from build123d import *

# Parameters (mm, degrees)
BOSS_EXTRUDE1_DEPTH = 5
SKETCH2_R           = 3
CUT_EXTRUDE1_DEPTH  = 5
CUT_EXTRUDE2_DEPTH  = 5
CUT_EXTRUDE7_DEPTH  = 5


with BuildPart() as part:
    # Sketch1 → Boss-Extrude1 (new body)
    with BuildSketch(Plane.XY):
        with BuildLine():
            Line((-0.6, -8), (-0.6, 192))
            Line((-0.6, 192), (11.4, 192))
            Line((11.4, 192), (11.4, -8))
            ThreePointArc((11.4, -8), (5.4, -14), (-0.6, -8))
        make_face()
    extrude(amount=BOSS_EXTRUDE1_DEPTH)

    # Sketch2 → Cut-Extrude1 (cut)
    with BuildSketch(Plane.XY.offset(5)):
        with Locations((5.4, -8)):
            Circle(SKETCH2_R)
    extrude(amount=-CUT_EXTRUDE1_DEPTH, mode=Mode.SUBTRACT)

    # Sketch4 → Cut-Extrude2 (cut)
    with BuildSketch(Plane.XY.offset(5)):
        with BuildLine():
            Line((2.4, 102), (2.4, 42))
            ThreePointArc((2.4, 42), (5.4, 39), (8.4, 42))
            Line((8.4, 42), (8.4, 102))
            ThreePointArc((8.4, 102), (5.4, 105), (2.4, 102))
        make_face()
    extrude(amount=-CUT_EXTRUDE2_DEPTH, mode=Mode.SUBTRACT)

    # Sketch5 → Cut-Extrude7 (cut)
    with BuildSketch(Plane.XY.offset(5)):
        with BuildLine():
            Line((2.4, 192), (2.4, 142))
            ThreePointArc((2.4, 142), (5.4, 139), (8.4, 142))
            Line((8.4, 142), (8.4, 192))
            Line((8.4, 192), (2.4, 192))
        make_face()
    extrude(amount=-CUT_EXTRUDE7_DEPTH, mode=Mode.SUBTRACT)


solid = part.part
Geometry: final body of the model. Coordinates: model frame, mm. A direction names the side the tool comes from. Give positions to 0.01 mm unless a question says otherwise; leave off trailing zeros. Write each loop counter-clockwise with the first axis right and the second up, starting at its lowest first coordinate (ties: lowest second). Pieces come first, ordered by that corner, then holes.
(1) Cut plane B-B, the plane x = 5.4. Return loops of the section in (y, z).
(2) Mould query, pull axis X, two halves, no side actions, for faces 1 (the flat face through (1, 90, 0)), 2 (the flat face through (2.4, 167, 3)), 3 (the flat face through (-0.6, 91, 2)), 4 (the cylindrical face through (5.3, 39, 2.5)). Classes: released by +X, released by -X, zero draft, split by the parting line, or undercut.
(3) First-contact query: P1, Ø1, axis at x = 3.5, z = 4, coming from the +Y side; P2, Ø6, axis at x = 4, y = 102, coming from the -Z side; P3, Ø1, axis at x = 9, z = 1.5, coming from the -Y side. Flat tips, straight axial feed; report the tip coordinate or a pass-through.
(4) Ray query, line 1 (Y direction, x = 5.5, z = 1.15); line 2 (X direction, y = 175, z = 3.1); line 3 (Y direction, x = 9.75, z = 2.8). Return the intervals inside material, ascending.
(5) Cut plane C-C, the plane z = 1.7. Return loops of the section in (x, y), then the cut area to 3 significant figures.
(6) Cut plane A-A, the plane y = 58. Return loops of the section in (x, z), then the cut area to 3 significant figures.
(7) Access query for faces 5 (the cylindrical face through (5.5, 105, 2.5)), 6 (the flat face through (8.4, 167, 3)), 7 (the cylindrical face through (5.5, -14, 2.5)). Directions: +Z, -Z, +X, -X, +Y, -Y. A direction counts if a zero-diameter tool reaches every point of the face in a straight line with its end or side. Return the directions, or none.
Values follow:
1. outline: (-14, 0) - (-11, 0) - (-11, 5) - (-14, 5) - close; (-5, 0) - (39, 0) - (39, 5) - (-5, 5) - close; (105, 0) - (139, 0) - (139, 5) - (105, 5) - close
2. face 1: zero draft
2. face 2: undercut
2. face 3: released by -X
2. face 4: undercut
3. P1: stops at y = 140.2
3. P2: stops at z = 0
3. P3: stops at y = -13.14
4. line 1: y = -14 to -11, -5 to 39, 105 to 139
4. line 2: x = -0.6 to 2.4, 8.4 to 11.4
4. line 3: y = -12.13 to 192
5. outline: (-0.6, -8) arc R6 ccw to (11.4, -8) - (11.4, 192) - (8.4, 192) - (8.4, 142) arc R3 cw to (2.4, 142) - (2.4, 192) - (-0.6, 192) - close; hole circle Ø6 at (5.4, -8); hole (2.4, 42) arc R3 ccw to (8.4, 42) - (8.4, 102) arc R3 ccw to (2.4, 102) - close
5. area: 1,730 mm2
6. outline: (-0.6, 0) - (2.4, 0) - (2.4, 5) - (-0.6, 5) - close; (8.4, 0) - (11.4, 0) - (11.4, 5) - (8.4, 5) - close
6. area: 30.0 mm2
7. face 5: +Z, -Z
7. face 6: +Z, -Z, +Y
7. face 7: +Z, -Z, -Y
